Here's how the part is built. I have some questions about the finished solid (model axes, mm). A direction names the side the tool comes from. Coordinates: 2 decimals unless noted, no trailing zeros. Loops run counter-clockwise (first coordinate to the right, second up) from the corner with the lowest first, then second, coordinate; pieces in that order, holes last. Notation, with made-up numbers: M 6,69.25 L 22,69.25 A25 cw 22,84.25 Z; hole C -7.5,-28.5 d1. An arc over 180 degrees is marked long. Use one line per item in the form item = value. Start each with the question number.
(1) Please list where these lines run through material, in increasing order: L1, parallel to Z at x = 0, y = -19; L2, parallel to Y at x = 7.5, z = 6; L3, parallel to X at y = -50, z = -5.
(2) Imagine slicing it at A-A, the plane z = 0. Please give me the cut outline in (x, y), and give its area (3 significant figures).
(3) Imagine slicing it at C-C, the plane y = -26. Please give me the cut outline in (x, z), and give its area (3 significant figures).
(4) Will these pins go through, and if not, where does the flat tip stop? P1, Ø3, axis at x = 4.5, y = -26, coming from the -Z side (3 decimals); P2, Ø2, axis at x = 1.5, y = -53.5, coming from the -Z side; P3, Ø3, axis at x = 12, y = -32.5, coming from the +Z side.
(5) Imagine slicing it at B-B, the plane x = 0. Please give me the cut outline in (y, z), and give its area (3 significant figures).
(6) On a 3-axis mill with a long thin cutter (end or side, diameter ignored), from which of +Z, -Z, +X, -X, +Y, -Y can I reach the whole of each face in a straight line? I mean faces 4 (the flat face through (0, -64, -15)), 5 (the flat face through (0, -3, 0)). Say none if no direction works.
(7) Thinking about a two-plate mould opening in X: for faces 1 (the cylindrical face through (6.691, -33.073, -12.864)), 2 (the flat face through (0, 0, 0)), 3 (the cylindrical face through (15.24, -32.57, -6.32)), which applies, +X half, -X half, draft (parallel to the pull), parting line (faces both ways), or undercut?
```python
from build123d import *

# Parameters (mm, degrees)
F0_R     = 16.5
F1_DEPTH = 3
F2_R     = 16.5
F2_R_2   = 14.5
F3_DEPTH = 61
F4_R     = 2


with BuildPart() as f1:
    # F0 (on Front) → F1 (new body)
    with BuildSketch(Plane.XZ):
        Circle(F0_R)
    extrude(amount=F1_DEPTH)

    # F2 (on face) → F3 (join)
    with BuildSketch(Plane.XZ.offset(3)):
        Circle(F2_R)
        Circle(F2_R_2, mode=Mode.SUBTRACT)
    extrude(amount=F3_DEPTH)

    # F4
    f4_edges = [f1.edges().sort_by_distance(p)[0] for p in [
        (-16.5, 0, 0),
    ]]
    fillet(f4_edges, radius=F4_R)


solid = f1.part
```
Answer:
q1.L1 = -16.5 to -14.5, 14.5 to 16.5
q1.L2 = -3 to 0
q1.L3 = -15.72 to -13.61, 13.61 to 15.72
q2.outline = M -16.5,-64 L -14.5,-64 L -14.5,-3 L 14.5,-3 L 14.5,-64 L 16.5,-64 L 16.5,-2 A2 ccw 14.5,0 L -14.5,0 A2 ccw -16.5,-2 Z
q2.area = 341 mm²
q3.outline = C 0,0 d33; hole C 0,0 d29
q3.area = 195 mm²
q4.P1 = -16.225
q4.P2 = -16.49
q4.P3 = 12.73
q5.outline = M -64,-16.5 L -2,-16.5 A2 ccw 0,-14.5 L 0,14.5 A2 ccw -2,16.5 L -64,16.5 L -64,14.5 L -3,14.5 L -3,-14.5 L -64,-14.5 Z
q5.area = 341 mm²
q6.face_4 = +Z, -Z, +X, -X, -Y
q6.face_5 = -Y
q7.face_1 = undercut
q7.face_2 = draft
q7.face_3 = parting line
